from build123d import *

# Parameters (mm, degrees)
BOSS_EXTRUDE1_DEPTH = 5
SKETCH3_R           = 2
CUT_EXTRUDE2_DEPTH  = 6


with BuildPart() as part:
    # Sketch1 → Boss-Extrude1 (new body)
    with BuildSketch(Plane.XY):
        with BuildLine():
            Line((0, -9), (0, 9))
            ThreePointArc((0, 9), (0.585786438, 10.414213562), (2, 11))
            Line((2, 11), (6, 11))
            ThreePointArc((6, 11), (7.414213562, 10.414213562), (8, 9))
            Line((8, 9), (8, -9))
            ThreePointArc((8, -9), (7.414213562, -10.414213562), (6, -11))
            Line((6, -11), (2, -11))
            ThreePointArc((2, -11), (0.585786438, -10.414213562), (0, -9))
        make_face()
    extrude(amount=BOSS_EXTRUDE1_DEPTH)

    # Sketch3 → Cut-Extrude2 (cut, through all)
    with BuildSketch(Plane.XY.offset(5)):
        with Locations((4, 0)):
            Circle(SKETCH3_R)
        with Locations((4, 8)):
            Circle(SKETCH3_R)
        with Locations((4, -8)):
            Circle(SKETCH3_R)
    extrude(amount=-CUT_EXTRUDE2_DEPTH, mode=Mode.SUBTRACT)


solid = part.part
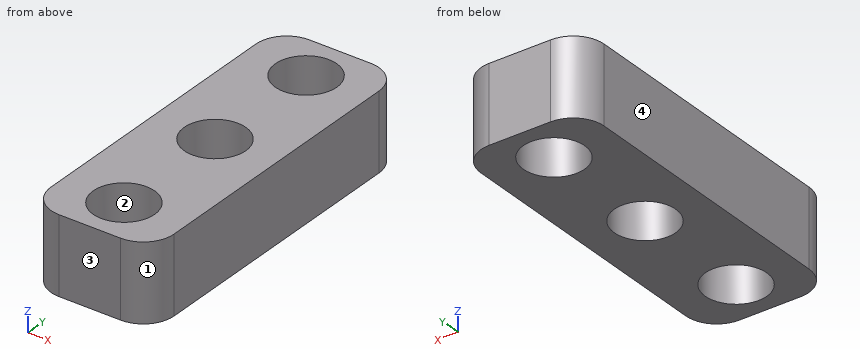
Check sheet for the modelled part. Datum: model origin and axes. Units: mm. Face numbers are marked on the shaded views. Round coordinates to 2 decimals unless told otherwise and drop trailing zeros. Loops run counter-clockwise (first coordinate to the right, second up) from the corner with the lowest first, then second, coordinate; pieces in that order, holes last.
1. Sectioned sample at B-B on y = -8. Record the boundary of the cut face in (x, z), and give its area (3 significant figures).
2. Mould release check, pull along X, two halves, no side actions. Record for the marked faces 1, 2, 3 and 4: released by +X, released by -X, zero draft, split by the parting line, or undercut.
3. Sectioned sample at A-A on x = 4. Record the boundary of the cut face in (y, z).
4. Sectioned sample at C-C on z = 1.95. Record the boundary of the cut face in (x, y), and give its area (3 significant figures).
5. Scan lines: probe 1 along Y at (x, z) = (4, 1.5); probe 2 along Y at (x, z) = (3.5, 1.2); probe 3 along X at (y, z) = (-7, 3.95). Record each from-to range of solid material in increasing order.
6. Gauge pin test, flat end, axial feed: pin 1 Ø2.5 at (x, y) = (4, 8) entering from +Z. Record the tip position at first contact, or that the pin passes through.
Recorded:
1. outline: (0, 0) - (2, 0) - (2, 5) - (0, 5) - close; (6, 0) - (8, 0) - (8, 5) - (6, 5) - close
1. area: 20.0 mm2
2. face 1: released by +X
2. face 2: undercut
2. face 3: zero draft
2. face 4: released by -X
3. outline: (-11, 0) - (-10, 0) - (-10, 5) - (-11, 5) - close; (-6, 0) - (-2, 0) - (-2, 5) - (-6, 5) - close; (2, 0) - (6, 0) - (6, 5) - (2, 5) - close; (10, 0) - (11, 0) - (11, 5) - (10, 5) - close
4. outline: (0, -9) arc R2 ccw to (2, -11) - (6, -11) arc R2 ccw to (8, -9) - (8, 9) arc R2 ccw to (6, 11) - (2, 11) arc R2 ccw to (0, 9) - close; hole circle Ø4 at (4, -8); hole circle Ø4 at (4, 0); hole circle Ø4 at (4, 8)
4. area: 135 mm2
5. probe 1: y = -11 to -10, -6 to -2, 2 to 6, 10 to 11
5. probe 2: y = -11 to -9.94, -6.06 to -1.94, 1.94 to 6.06, 9.94 to 11
5. probe 3: x = 0 to 2.27, 5.73 to 8
6. pin 1: passes through
